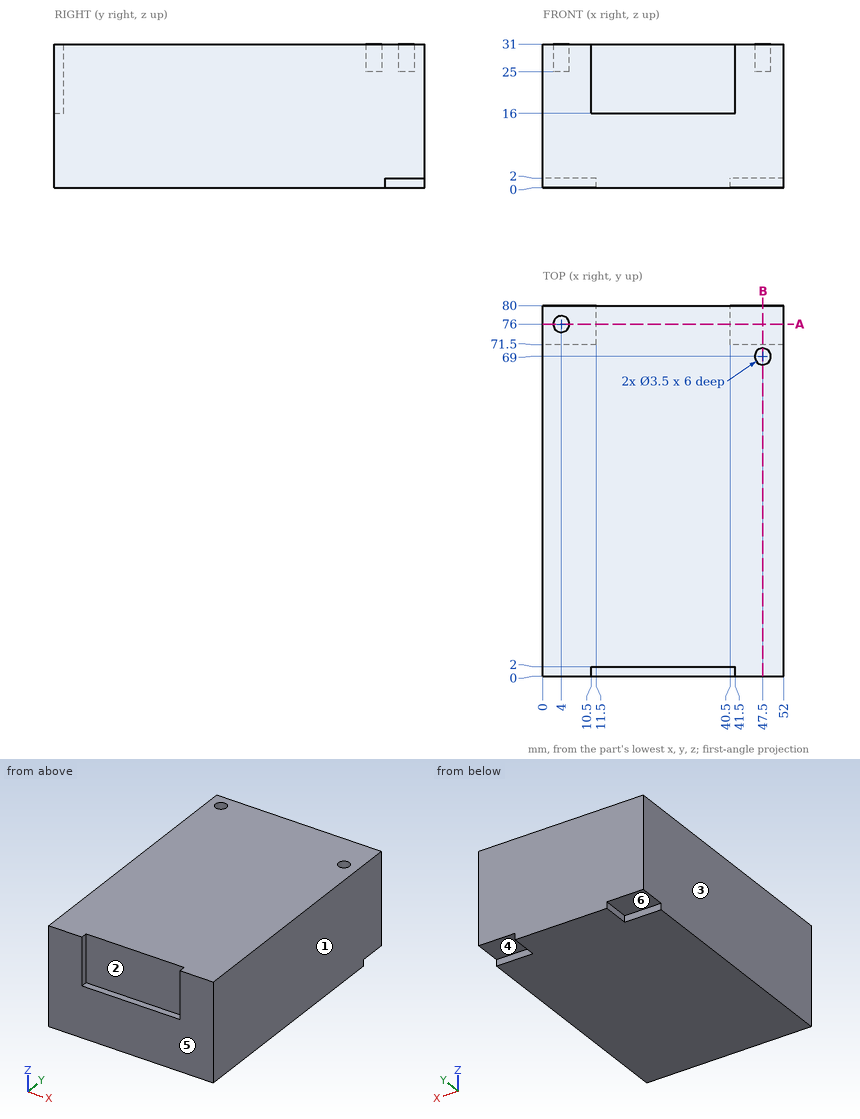
Input: dimensioned drawing with shaded views. Units: mm. Origin: part minimum x, y, z. A direction names the side the tool comes from. Round coordinates to 2 decimals unless told otherwise and drop trailing zeros. Order: outer loops, then holes, each group sorted by start corner. A loop starts at its lowest first (then second) coordinate and runs counter-clockwise, first axis right, second up. Notation, with made-up numbers: (41.25, 66) - (68.25, 66) arc R25 cw to (68.25, 92) - close; hole circle Ø8 at (78.25, -23.5). An arc over 180 degrees is marked (long way). Answer as a JSON object with one key per item and string values. Group by question number.
(1) Draft query along X for the marked faces 1, 2, 3 and 4. Return one class per face: released by +X, released by -X, zero draft, split by the parting line, or undercut.
(2) Pin query (flat end, axial travel): P1, Ø0.6, axis at x = 43.5, z = 1, coming from the +Y side; P2, Ø1.6, axis at y = 74, z = 0.5, coming from the +X side; P3, Ø1.8, axis at x = 48, y = 69.5, coming from the +Z side. Return the tip coordinate at first contact, or that it passes through.
(3) Reachability of the marked faces 5 and 6 from +Z, -Z, +X, -X, +Y, -Y: full face, straight path, thin tool, end or side. Return the list, or none.
(4) Cut plane B-B (x = 47.5). Return loops of the section in (y, z).
(5) Cut plane A-A (y = 76). Return loops of the section in (x, z).
(6) Material intervals for probe 1 along Y at (x, z) = (47.5, 29.75); probe 2 along X at (y, z) = (69, 28.6); probe 3 along Y at (x, z) = (4, 28), sorted ascending. Write a range as from..to.
Here are the results:
{
 "1": {"face 1": "released by +X", "face 2": "undercut", "face 3": "released by -X", "face 4": "zero draft"},
 "2": {"P1": "stops at y = 71.5", "P2": "stops at x = 40.5", "P3": "stops at z = 25"},
 "3": {"face 5": "+Z, -Z, +X, -X, -Y", "face 6": "-Z, -X, +Y"},
 "4": {"outline": "(0, 0) - (71.5, 0) - (71.5, 2) - (80, 2) - (80, 31) - (70.75, 31) - (70.75, 25) - (67.25, 25) - (67.25, 31) - (0, 31) - close"},
 "5": {"outline": "(0, 2) - (11.5, 2) - (11.5, 0) - (40.5, 0) - (40.5, 2) - (52, 2) - (52, 31) - (5.75, 31) - (5.75, 25) - (2.25, 25) - (2.25, 31) - (0, 31) - close"},
 "6": {"probe 1": "y = 0..67.25, 70.75..80", "probe 2": "x = 0..45.75, 49.25..52", "probe 3": "y = 0..74.25, 77.75..80"}
}
